from build123d import *

# Parameters (mm, degrees)
SKETCH2_R           = 47.6885
BOSS_EXTRUDE1_DEPTH = 57.658
SKETCH5_R           = 2.54
SKETCH5_R_2         = 5.6388
CUT_EXTRUDE2_DEPTH  = 89.728975135
SKETCH4_R           = 3.175
CUT_EXTRUDE3_DEPTH  = 89.728975135
CUT_EXTRUDE4_DEPTH  = 43.18
SKETCH11_R          = 6.35
CUT_EXTRUDE7_DEPTH  = 7.62
SKETCH14_R          = 2.067000057
CUT_EXTRUDE8_DEPTH  = 19.05
SKETCH15_R          = 2.38125
CUT_EXTRUDE9_DEPTH  = 66.04


with BuildPart() as part:
    # Sketch2 → Boss-Extrude1 (new body)
    with BuildSketch(Plane(origin=(0, 0, 0), x_dir=(1, 0, 0), z_dir=(0, 1, 0))):
        with Locations(Location((0, 0, 0), (0, 0, 90))):
            Circle(SKETCH2_R)
    extrude(amount=BOSS_EXTRUDE1_DEPTH)

    # Sketch5 → Cut-Extrude2 (cut, through all)
    with BuildSketch(Plane(origin=(0, 57.658, 0), x_dir=(1, 0, 0), z_dir=(0, 1, 0))):
        with Locations(Location((-41.445499463, 16.673368884, 0), (0, 0, 270))):
            Circle(SKETCH5_R)
        with Locations(Location((-44.648658026, 1.492646038, 0), (0, 0, 270))):
            Circle(SKETCH5_R)
        with Locations(Location((-42.466529486, -13.86811195, 0), (0, 0, 270))):
            Circle(SKETCH5_R)
        with Locations(Location((-30.694251769, -25.755535339, 0), (0, 0, 270))):
            Circle(SKETCH5_R_2)
    extrude(amount=-CUT_EXTRUDE2_DEPTH, mode=Mode.SUBTRACT)

    # Sketch4 → Cut-Extrude3 (cut, through all)
    with BuildSketch(Plane(origin=(0, 57.658, 0), x_dir=(1, 0, 0), z_dir=(0, 1, 0))):
        with Locations(Location((-26.162, 0, 0), (0, 0, 270))):
            Circle(SKETCH4_R)
        with Locations(Location((26.162, 0, 0), (0, 0, 270))):
            Circle(SKETCH4_R)
        with Locations(Location((0, 26.162, 0), (0, 0, 270))):
            Circle(SKETCH4_R)
        with Locations(Location((0, -26.162, 0), (0, 0, 270))):
            Circle(SKETCH4_R)
    extrude(amount=-CUT_EXTRUDE3_DEPTH, mode=Mode.SUBTRACT)

    # Sketch6 → Cut-Extrude4 (cut)
    with BuildSketch(Plane(origin=(0, 57.658, 0), x_dir=(1, 0, 0), z_dir=(0, 1, 0))):
        Polygon((-27.050344847, -30.987270671), (20.620600848, 9.013402279), (12.457198205, 18.742166707), (-35.21374749, -21.258506244), align=None)
    extrude(amount=-CUT_EXTRUDE4_DEPTH, mode=Mode.SUBTRACT)

    # Sketch11 → Cut-Extrude7 (cut)
    with BuildSketch(Plane.XZ):
        with Locations(Location((0, 26.162, 0), (0, 0, 270))):
            Circle(SKETCH11_R)
        with Locations(Location((26.162, 0, 0), (0, 0, 270))):
            Circle(SKETCH11_R)
        with Locations(Location((0, -26.162, 0), (0, 0, 270))):
            Circle(SKETCH11_R)
        with Locations(Location((-26.162, 0, 0), (0, 0, 270))):
            Circle(SKETCH11_R)
    extrude(amount=-CUT_EXTRUDE7_DEPTH, mode=Mode.SUBTRACT)

    # Sketch14 → Cut-Extrude8 (cut)
    with BuildSketch(Plane.XZ):
        with Locations(Location((1.356935186, -14.949033782, 0), (0, 0, 270))):
            Circle(SKETCH14_R)
        with Locations(Location((4.523691953, 8.972265338, 0), (0, 0, 270))):
            Circle(SKETCH14_R)
    extrude(amount=-CUT_EXTRUDE8_DEPTH, mode=Mode.SUBTRACT)

    # Sketch15 → Cut-Extrude9 (cut)
    with BuildSketch(Plane.XZ):
        with Locations(Location((31.589006405, 31.589006405, 0), (0, 0, 270))):
            Circle(SKETCH15_R)
    extrude(amount=-CUT_EXTRUDE9_DEPTH, mode=Mode.SUBTRACT)


solid = part.part
Verification items for the finished model (mm, model axes). A direction names the side the tool comes from. Coordinates: 2 decimals unless noted, no trailing zeros. Loops run counter-clockwise (first coordinate to the right, second up) from the corner with the lowest first, then second, coordinate; pieces in that order, holes last. Notation, with made-up numbers: (-5, 0.25) -> (38, 0.25) arc R31 cw to (38, 35.25) -> close; hole circle Ø6 at (-30.5, 64). An arc over 180 degrees is marked (long way). Answer as a JSON object with one key per item and string values. Group by question number.
Item 1: Sectioned sample at A-A on z = -1. Record the boundary of the cut face in (x, y), plus the area to 3 significant figures.
Item 2: Scan lines: probe 1 along Z at (x, y) = (-1, 49); probe 2 along X at (y, z) = (44, 0); probe 3 along X at (y, z) = (17.5, 16). Record each from-to range of solid material in increasing order.
Item 3: Mould release check, pull along Z, two halves, no side actions. Record for faces 1 (the cylindrical face through (0.14, 32.989, -29.334)), 2 (the flat face through (-1, 57.658, -10)): +Z half, -Z half, draft (parallel to the pull), parting line (faces both ways), or undercut.
Item 4: Tool access check on faces 3 (the flat face through (28, 7.62, 3)), 4 (the flat face through (-11.045, 36.37, 0.978)), 5 (the cylindrical face through (31.69, 28.43, 33.97)). Record the directions out of +Z, -Z, +X, -X, +Y, -Y that give a thin tool (end or side, any length) a straight path to the whole face; none if there is none.
Item 5: Sectioned sample at B-B on y = 17.5. State how many separate pieces and enclosed holes the cut face has, plus the area to 3 significant figures.
Item 6: Depth check by flat-ended pin: pin 1 (11.5 mm diameter, centred on x = 0, z = 26.162, fed in from -Y); pin 2 (3 mm diameter, centred on x = 11.5, y = 17, fed in from -Z); pin 3 (8 mm diameter, centred on x = 11, y = 6.5, fed in from -Z). Enter the tip coordinate at first touch or a pass-through.
Evaluation:
{
 "1": {"outline": "(-47.68, 0) -> (-47.14, 0) -> (-47.14, 57.66) -> (-47.68, 57.66) -> close; (-42.16, 0) -> (-32.43, 0) -> (-32.43, 7.62) -> (-29.18, 7.62) -> (-29.18, 57.66) -> (-42.16, 57.66) -> close; (-23.15, 7.62) -> (-19.89, 7.62) -> (-19.89, 0) -> (19.89, 0) -> (19.89, 7.62) -> (23.15, 7.62) -> (23.15, 57.66) -> (11.07, 57.66) -> (11.07, 14.48) -> (-8.69, 14.48) -> (-8.69, 57.66) -> (-23.15, 57.66) -> close; (29.18, 7.62) -> (32.43, 7.62) -> (32.43, 0) -> (47.68, 0) -> (47.68, 57.66) -> (29.18, 57.66) -> close", "area": "3,560 mm²"},
 "2": {"probe 1": "z = -47.68 to -29.18, -23.15 to -7.45, 9.13 to 23.15, 29.18 to 47.68", "probe 2": "x = -47.69 to -46.7, -42.59 to -29.34, -22.99 to -9.88, 9.88 to 22.99, 29.34 to 47.69", "probe 3": "x = -44.92 to -43.85, -41.09 to -28.95, -9.19 to 44.92"},
 "3": {"face 1": "undercut", "face 2": "draft"},
 "4": {"face 3": "-Y", "face 4": "+Y", "face 5": "+Y, -Y"},
 "5": {"separate pieces": "1", "enclosed holes": "11", "area": "6,080 mm²"},
 "6": {"pin 1": "stops at y = 7.62", "pin 2": "stops at z = -46.63", "pin 3": "stops at z = -47.17"}
}
